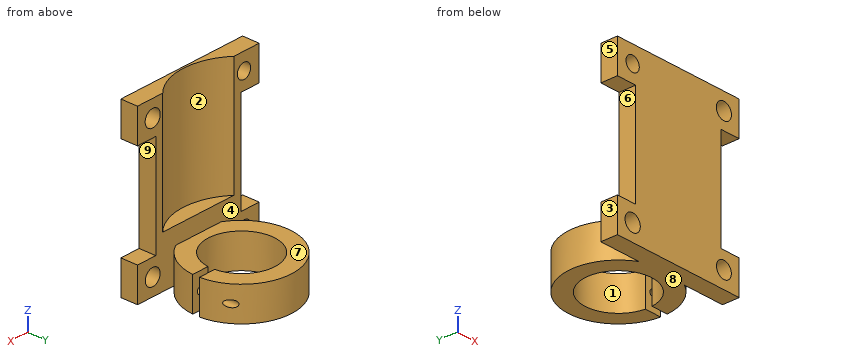
from build123d import *

# Parameters (mm, degrees)
SKETCH1_W               = 6
SKETCH1_H               = 10
SKETCH1_W_2             = 28
SKETCH1_H_2             = 50
BOSS_EXTRUDE1_DEPTH     = 5
BOSS_EXTRUDE2_DEPTH     = 10
SKETCH4_R               = 17.5
CUT_EXTRUDE1_DEPTH      = 35
CUT_EXTRUDE2_DEPTH      = 30
CUT_EXTRUDE2_DEPTH_BACK = 5
SKETCH6_R               = 1
SKETCH5_R               = 2.179957699
SKETCH5_R_2             = 2.482189609
SKETCH5_R_3             = 2.446214892
SKETCH5_R_4             = 2.511545909
CUT_EXTRUDE3_DEPTH      = 30


with BuildPart() as part:
    # Sketch1 → Boss-Extrude1 (new body)
    with BuildSketch(Plane(origin=(0, 0, 0), x_dir=(1, 0, 0), z_dir=(0, 1, 0))):
        with Locations((-17, -20)):
            Rectangle(SKETCH1_W, SKETCH1_H)
        Rectangle(SKETCH1_W_2, SKETCH1_H_2)
        with Locations((-17, 20)):
            Rectangle(SKETCH1_W, SKETCH1_H)
        with Locations((17, 20)):
            Rectangle(SKETCH1_W, SKETCH1_H)
        with Locations((17, -20)):
            Rectangle(SKETCH1_W, SKETCH1_H)
    extrude(amount=BOSS_EXTRUDE1_DEPTH)

    # Sketch2 → Boss-Extrude2 (add)
    with BuildSketch(Plane(origin=(0, 0, -25), x_dir=(-1, 0, 0), z_dir=(0, 0, -1))):
        with BuildLine():
            Line((-9.949874371, 19), (-14.966629547, 19))
            ThreePointArc((-14.966629547, 19), (15, 18), (-14.966629547, 17))
            Line((-14.966629547, 17), (-9.949874371, 17))
            ThreePointArc((-9.949874371, 17), (10, 18), (-9.949874371, 19))
        make_face()
    extrude(amount=-BOSS_EXTRUDE2_DEPTH)

    # Sketch4 → Cut-Extrude1 (cut)
    with BuildSketch(Plane.XY.offset(25)):
        with Locations((0, 18)):
            Circle(SKETCH4_R)
    extrude(amount=-CUT_EXTRUDE1_DEPTH, mode=Mode.SUBTRACT)

    # Sketch6 → Cut-Extrude2 (cut, two sides: drawn at the far end of the back side and taken through both)
    with BuildSketch(Plane(origin=(0, 17, 0), x_dir=(1, 0, 0), z_dir=(0, 1, 0)).offset(-CUT_EXTRUDE2_DEPTH_BACK)):
        with Locations(Location((12.458251959, 20, 0), (0, 0, 180))):
            Circle(SKETCH6_R)
    extrude(amount=CUT_EXTRUDE2_DEPTH + CUT_EXTRUDE2_DEPTH_BACK, mode=Mode.SUBTRACT)

    # Sketch5 → Cut-Extrude3 (cut)
    with BuildSketch(Plane(origin=(0, 5, 0), x_dir=(1, 0, 0), z_dir=(0, 1, 0))):
        with Locations(Location((-15, -20, 0), (0, 0, 270))):
            Circle(SKETCH5_R)
        with Locations(Location((15, -20, 0), (0, 0, 270))):
            Circle(SKETCH5_R_2)
        with Locations(Location((15, 20, 0), (0, 0, 270))):
            Circle(SKETCH5_R_3)
        with Locations(Location((-15, 20, 0), (0, 0, 270))):
            Circle(SKETCH5_R_4)
    extrude(amount=-CUT_EXTRUDE3_DEPTH, mode=Mode.SUBTRACT)


solid = part.part
Geometry check sheet. Reference: the model listing, model coordinates, mm. Face numbers are marked on the shaded views. A direction names the side the tool comes from. Round coordinates to 2 decimals unless told otherwise and drop trailing zeros. Loops run counter-clockwise (first coordinate to the right, second up) from the corner with the lowest first, then second, coordinate; pieces in that order, holes last.
Item 1: Access from +Z, -Z, +X, -X, +Y, -Y to the whole of each face (thin tool, end or side, straight path). Record for the marked faces 5, 6, 7, 8 and 9.
Item 2: Gauge pin test, flat ends, axial feed: pin 1 (4 mm diameter, centred on x = -9.5, z = 16.5, fed in from -Y); pin 2 (2.5 mm diameter, centred on x = -1.5, y = 2.5, fed in from +Z); pin 3 (1 mm diameter, centred on y = 16, z = -17, fed in from +X); pin 4 (1.8 mm diameter, centred on x = 12.46, z = -20, fed in from +Y). Record the tip position at first contact, or that the pin passes through.
Item 3: Mould release check, pull along Y, two halves, no side actions. Record for the marked faces 1, 2, 3 and 4: pulls with the +Y half, pulls with the -Y half, needs draft (parallel to the pull), parting line crosses it, or undercut.
Item 4: Cross-section at C-C on x = 5. Record the boundary of the cut face in (y, z).
Item 5: Cross-section at B-B on z = 20. Record the boundary of the cut face in (x, y).
Item 6: Cross-section at D-D on z = -20. Record the boundary of the cut face in (x, y).
Item 7: Cross-section at A-A on y = 15.5. Record the boundary of the cut face in (x, z).
Item 8: Thickness scan on line 1 (X direction, y = 2.7, z = -20); line 2 (Y direction, x = 12.5, z = -22); line 3 (Y direction, x = 0, z = -18). Record the ranges inside material, lowest first.
Answer sheet:
1. face 5: +Z, -Z, -X, +Y, -Y
1. face 6: -X, +Y, -Y
1. face 7: +Z, +X, -X, +Y
1. face 8: -Z, +X, -X, +Y, -Y
1. face 9: +X, +Y, -Y
2. pin 1: stops at y = 0
2. pin 2: stops at z = -10
2. pin 3: stops at x = 14.92
2. pin 4: stops at y = 12
3. face 1: undercut
3. face 2: pulls with the +Y half
3. face 3: needs draft
3. face 4: undercut
4. outline: (0, -25) - (9.34, -25) - (9.34, -15) - (5, -15) - (5, -10) - (1.23, -10) - (1.23, 25) - (0, 25) - close; (26.66, -25) - (32.14, -25) - (32.14, -15) - (26.66, -15) - close
5. outline: (-20, 0) - (-17.18, 0) - (-17.18, 5) - (-20, 5) - close; (-12.82, 0) - (12.52, 0) - (12.52, 5) - (11.72, 5) arc R17.5 cw to (-11.72, 5) - (-12.82, 5) - close; (17.48, 0) - (20, 0) - (20, 5) - (17.48, 5) - close
6. outline: (-20, 0) - (-17.51, 0) - (-17.51, 5) - (-20, 5) - close; (-12.49, 0) - (12.55, 0) - (12.55, 5) - (7.48, 5) arc R15 ccw to (14.97, 17) - (13.46, 17) - (13.46, 12) - (11.46, 12) - (11.46, 17) - (9.95, 17) arc R10 cw (long way) to (9.95, 19) - (11.46, 19) - (11.46, 27.68) arc R15 ccw (long way) to (-7.48, 5) - (-12.49, 5) - close; (13.46, 19) - (14.97, 19) arc R15 ccw to (13.46, 24.62) - close; (17.45, 0) - (20, 0) - (20, 5) - (17.45, 5) - close
7. outline: (-14.79, -25) - (-9.68, -25) - (-9.68, -15) - (-14.79, -15) - close; (9.68, -25) - (14.79, -25) - (14.79, -15) - (9.68, -15) - close; hole circle Ø2 at (12.46, -20)
8. line 1: x = -20 to -17.51, -12.49 to 12.55, 17.45 to 20
8. line 2: y = 0 to 5, 9.71 to 17, 19 to 26.29
8. line 3: y = 0 to 8, 28 to 33
